Part model, mm, in its own coordinate system. A direction names the side the tool comes from. Coordinates: 2 decimals unless noted, no trailing zeros. Loops run counter-clockwise (first coordinate to the right, second up) from the corner with the lowest first, then second, coordinate; pieces in that order, holes last. Notation, with made-up numbers: M -0.75,2.25 L 26.25,2.25 A26 cw 26.25,24.25 Z; hole C -10,8 d2. An arc over 180 degrees is marked long. Answer as a JSON object with one key per item and string values. Group by question number.
1. Saw through at B-B on y = -5. Write the cut outline in (x, z).
2. Saw through at D-D on x = -3. Write the cut outline in (y, z).
3. Saw through at A-A on z = 22. Write the cut outline in (x, y), then the cut area to 3 significant figures.
4. Drill centre lines: L1, parallel to X at y = 10, z = 49.5; L2, parallel to Y at x = -8, z = 27; L3, parallel to X at y = -5, z = 47. Where is each one in solid material? Low to high.
5. Mould opens along Z. For faces 1 (the face through (23.613, 8, 39)), 2 (the face through (4.035, 0.068, 12.491)), 3 (the face through (2.88, -6.27, 24.04)) say: released by +Z, released by -Z, zero draft, split by the parting line, or undercut.
6. Drop flat-ended pins along their axis: pin 1 Ø4 at (x, y) = (-6, -2) entering from -Z; pin 2 Ø20 at (x, z) = (7.5, 41.5) entering from +Y; pin 3 Ø10 at (x, y) = (-1.5, 10) entering from +Z. Give the stop position or say it passes through.
7. 3-axis set-ups, long thin cutter, end or side, ignore diameter. For faces 4 (the face through (9.829, -6.265, 46.918)), 5 (the face through (51.87, 0, 38)), 6 (the face through (-16.062, 8, 39)): which of +Z, -Z, +X, -X, +Y, -Y reach the whole face in a straight line?
8. Saw through at C-C on z = 29. Write the cut outline in (x, y), then the cut area to 3 significant figures.
from build123d import *

# Parameters (mm, degrees)
F0_W     = 97.028
F0_H     = 29.2862
F2_DEPTH = 63.5
F1_W     = 39.6748
F1_H     = 12.0142
F3_DEPTH = 63.5
F5_DEPTH = 97.028
F6_R     = 3.2385
F7_DEPTH = 25.4
F9_DEPTH = 25.4


with BuildPart() as f2:
    # F0 (on Top) → F2 (new body)
    with BuildSketch(Plane.XY):
        with Locations((3.356052, -0.137089)):
            Rectangle(F0_W, F0_H)
    extrude(amount=F2_DEPTH)

    # F1 (on face) → F3 (cut)
    with BuildSketch(Plane.XY):
        with Locations((3.775152, 8.498911)):
            Rectangle(F1_W, F1_H)
    extrude(amount=F3_DEPTH, mode=Mode.SUBTRACT)

    # F4 (on face) → F5 (cut)
    with BuildSketch(Plane.YZ.offset(51.870052)):
        Polygon((14.506011, 0), (14.506011, 24.638), (-14.780189, 0), align=None)
    extrude(amount=-F5_DEPTH, mode=Mode.SUBTRACT)

    # F6 (on face) → F7 (cut)
    with BuildSketch(Plane.XZ.offset(14.780189)):
        with Locations((3.305252, 20.828)):
            Circle(F6_R)
    extrude(amount=-F7_DEPTH, mode=Mode.SUBTRACT)

    # F8 (on face) → F9 (cut)
    with BuildSketch(Plane.XZ.offset(14.780189)):
        Polygon((17.332412, 42.000698), (3.790186, 55.542924), (-5.854609, 45.898129), (-4.561452, 44.604972), (3.790186, 52.95661), (16.039255, 40.707541), align=None)
    extrude(amount=-F9_DEPTH, mode=Mode.SUBTRACT)


solid = f2.part
Outcome:
{
 "1": {"outline": "M -45.16,8.23 L 51.87,8.23 L 51.87,63.5 L -45.16,63.5 Z; hole M -5.85,45.9 L -4.56,44.6 L 3.79,52.96 L 16.04,40.71 L 17.33,42 L 3.79,55.54 Z; hole C 3.31,20.83 d6.48"},
 "2": {"outline": "M -14.78,0 L 2.49,14.53 L 2.49,46.17 L -14.78,46.17 Z; M -14.78,48.75 L 2.49,48.75 L 2.49,63.5 L -14.78,63.5 Z"},
 "3": {"outline": "M -45.16,-14.78 L 0.29,-14.78 L 0.29,2.49 L -16.06,2.49 L -16.06,11.37 L -45.16,11.37 Z; M 6.32,-14.78 L 51.87,-14.78 L 51.87,11.37 L 23.61,11.37 L 23.61,2.49 L 6.32,2.49 Z", "area": "2,080 mm²"},
 "4": {"L1": "x = -45.16 to -16.06, 23.61 to 51.87", "L2": "y = -14.78 to 2.49", "L3": "x = -45.16 to -4.75, -2.17 to 9.75, 12.33 to 51.87"},
 "5": {"face 1": "zero draft", "face 2": "released by -Z", "face 3": "undercut"},
 "6": {"pin 1": "stops at z = 9.07", "pin 2": "stops at y = 2.49", "pin 3": "passes through"},
 "7": {"face 4": "+Y, -Y", "face 5": "+Z, -Z, +X, +Y, -Y", "face 6": "+Z, -Z, +Y"},
 "8": {"outline": "M -45.16,-14.78 L 51.87,-14.78 L 51.87,14.51 L 23.61,14.51 L 23.61,2.49 L -16.06,2.49 L -16.06,14.51 L -45.16,14.51 Z", "area": "2,360 mm²"}
}
